The listing builds one solid part. Answer for the finished solid, in the listing's coordinates (mm). A direction names the side the tool comes from. Round coordinates to 2 decimals unless told otherwise and drop trailing zeros. Order: outer loops, then holes, each group sorted by start corner. A loop starts at its lowest first (then second) coordinate and runs counter-clockwise, first axis right, second up. Notation, with made-up numbers: (60.25, 46.5) - (119.25, 46.5) arc R23 cw to (119.25, 61.5) - close; hole circle Ø7 at (43.5, -26). An arc over 180 degrees is marked (long way). Write item = value, one per line.
from build123d import *

# Parameters (mm, degrees)
SKETCH1_R               = 15.5
BOSS_EXTRUDE2_DEPTH     = 2.5
SKETCH2_R               = 12.5
CUT_EXTRUDE1_DEPTH      = 1
BOSS_EXTRUDE3_DEPTH     = 9
SKETCH4_R               = 7
CUT_EXTRUDE2_DEPTH      = 1
CUT_EXTRUDE2_DEPTH_BACK = 12.5


with BuildPart() as part:
    # Sketch1 → Boss-Extrude2 (new body)
    with BuildSketch(Plane(origin=(0, 0, 0), x_dir=(0, 0, -1), z_dir=(1, 0, 0))):
        Circle(SKETCH1_R)
    extrude(amount=BOSS_EXTRUDE2_DEPTH)

    # Sketch2 → Cut-Extrude1 (cut)
    with BuildSketch(Plane(origin=(2.5, 0, 0), x_dir=(0, 0, -1), z_dir=(1, 0, 0))):
        Circle(SKETCH2_R)
    extrude(amount=-CUT_EXTRUDE1_DEPTH, mode=Mode.SUBTRACT)

    # Sketch3 → Boss-Extrude3 (add)
    with BuildSketch(Plane.ZY):
        Polygon((12.124355653, 0), (6.062177826, 10.5), (-6.062177826, 10.5), (-12.124355653, 0), (-6.062177826, -10.5), (6.062177826, -10.5), align=None)
    extrude(amount=BOSS_EXTRUDE3_DEPTH)

    # Sketch4 → Cut-Extrude2 (cut, two sides)
    with BuildSketch(Plane.ZY.offset(9)) as cut_extrude2_sk:
        Circle(SKETCH4_R)
    extrude(amount=CUT_EXTRUDE2_DEPTH, mode=Mode.SUBTRACT)
    extrude(cut_extrude2_sk.sketch, amount=-CUT_EXTRUDE2_DEPTH_BACK, mode=Mode.SUBTRACT)


solid = part.part
Q1. Determine the mould class of faces 4 (the face through (-3.824, -2.681, 6.466)), 5 (the face through (1.5, -5.4, -5.4)), 6 (the face through (-4, -10.5, 0)), 7 (the face through (1.232, 15.368, 2.018)) for opening direction Y: released by +Y, released by -Y, zero draft, split by the parting line, or undercut.
Model answer:
face_4 = undercut
face_5 = undercut
face_6 = released by -Y
face_7 = split by the parting line
Q2. Flat-ended cylindrical pins translate along their axes: P1, Ø2, axis at x = -7, z = 2.5, coming from the -Y side; P2, Ø1.5, axis at y = 0, z = 7.5, coming from the +X side; P3, Ø2, axis at x = -3, y = -10, coming from the +Z side; P4, Ø12.5, axis at y = 0, z = 0, coming from the -X side. Find the tip coordinate at first contact, or state that the pin passes through.
Model answer:
P1 = -10.5
P2 = 1.5
P3 = 6.93
P4 = through
Q3. Section A-A on x = -6.5 is taken. Determine the outline of the cut face in (y, z).
Model answer:
outline = (-10.5, -6.06) - (0, -12.12) - (10.5, -6.06) - (10.5, 6.06) - (0, 12.12) - (-10.5, 6.06) - close; hole circle Ø14 at (0, 0)
Q4. Section C-C on y = 7.5 is taken. Determine the outline of the cut face in (x, z).
Model answer:
outline = (-9, -7.79) - (0, -7.79) - (0, -13.56) - (2.5, -13.56) - (2.5, -10) - (1.5, -10) - (1.5, 10) - (2.5, 10) - (2.5, 13.56) - (0, 13.56) - (0, 7.79) - (-9, 7.79) - close
Q5. Find the intervals of material crossed by line 1 (Y direction, x = 1.75, z = 0); line 2 (X direction, y = -5, z = -7); line 3 (Z direction, x = -3.5, y = 6), in increasing order. Write a range as from..to.
Model answer:
line_1 = -15.5..-12.5, 12.5..15.5
line_2 = -9..1.5
line_3 = -8.66..-3.61, 3.61..8.66
Q6. Section D-D on z = 11.5 is taken. Determine the outline of the cut face in (x, y).
Model answer:
outline = (-9, -1.08) - (0, -1.08) - (0, -10.39) - (2.5, -10.39) - (2.5, -4.9) - (1.5, -4.9) - (1.5, 4.9) - (2.5, 4.9) - (2.5, 10.39) - (0, 10.39) - (0, 1.08) - (-9, 1.08) - close
Q7. Section B-B on z = 0 is taken. Determine the outline of the cut face in (x, y), then the cut area to 3 significant figures.
Model answer:
outline = (-9, -10.5) - (0, -10.5) - (0, -15.5) - (2.5, -15.5) - (2.5, -12.5) - (1.5, -12.5) - (1.5, -7) - (-9, -7) - close; (-9, 7) - (1.5, 7) - (1.5, 12.5) - (2.5, 12.5) - (2.5, 15.5) - (0, 15.5) - (0, 10.5) - (-9, 10.5) - close
area = 94.5 mm^2
Q8. For faces 1 (the face through (-4.437, -5.324, 9.051)), 2 (the face through (-4.437, 5.176, 9.136)), 3 (the face through (-4.437, 5.324, -9.051)), determine the directions among +Z, -Z, +X, -X, +Y, -Y from which every point of the face is accessible in a straight line to the end or side of a thin tool.
Model answer:
face_1 = +Z, -X, -Y
face_2 = +Z, -X, +Y
face_3 = -Z, -X, +Y
